Input: part model. Units: mm. Frame: model coordinates. A direction names the side the tool comes from. Coordinates: 2 decimals unless noted, no trailing zeros. Write each loop counter-clockwise with the first axis right and the second up, starting at its lowest first coordinate (ties: lowest second). Pieces come first, ordered by that corner, then holes.
from build123d import *

# Parameters (mm, degrees)
F1_DEPTH = 38.1
F3_DEPTH = 25
F5_R     = 4.7625
F6_DEPTH = 34.1
F8_DEPTH = 34.1
F9_DEPTH = 50


with BuildPart() as f1:
    # F0 (on Top) → F1 (new body)
    with BuildSketch(Plane.XY):
        Polygon((23.88, 22.062646), (-14.22, 22.062646), (-14.22, 3.012646), (-14.22, -16.037354), (23.88, -16.037354), align=None)
        with BuildLine():
            ThreePointArc((9.5925, 3.012646), (4.83, -1.749854), (0.0675, 3.012646))
            ThreePointArc((0.0675, 3.012646), (4.83, 7.775146), (9.5925, 3.012646))
        make_face(mode=Mode.SUBTRACT)
    extrude(amount=F1_DEPTH)

    # F2 (on face) → F3 (cut)
    with BuildSketch(Plane.YZ.offset(23.88)):
        with BuildLine():
            ThreePointArc((-1.749854, 19.05), (3.012646, 14.2875), (7.775146, 19.05))
            ThreePointArc((7.775146, 19.05), (3.012646, 23.8125), (-1.749854, 19.05))
        make_face()
    extrude(amount=-F3_DEPTH, mode=Mode.SUBTRACT)

    # F5 (on face) → F6 (cut)
    with BuildSketch(Plane.XY.offset(38.1)):
        Polygon((19.88, 18.062646), (4.83, 18.062646), (-10.22, 18.062646), (-10.22, 3.012646), (-10.22, -12.037354), (4.83, -12.037354), (19.88, -12.037354), (19.88, 3.012646), align=None)
        with Locations((4.83, 3.012646)):
            Circle(F5_R, mode=Mode.SUBTRACT)
    extrude(amount=-F6_DEPTH, mode=Mode.SUBTRACT)

    # F7 (on face) → F8 (cut)
    with BuildSketch(Plane(origin=(-14.22, 0, 0), x_dir=(0, -1, 0), z_dir=(-1, 0, 0))):
        Polygon((12.037354, 34.1), (-3.012646, 34.1), (-18.062646, 34.1), (-18.062646, 19.05), (-18.062646, 4), (-3.012646, 4), (12.037354, 4), (12.037354, 19.05), align=None)
    extrude(amount=-F8_DEPTH, mode=Mode.SUBTRACT)

    # F4 (on face) → F9 (cut)
    with BuildSketch(Plane.XZ.offset(16.037354)):
        Polygon((-14.22, 0), (23.88, 38.1), (-14.22, 38.1), align=None)
    extrude(amount=-F9_DEPTH, mode=Mode.SUBTRACT)


solid = f1.part
Item 1: Section query C-C, the plane z = 8.5. Return loops of the section in (x, y).
Item 2: Section query B-B, the plane x = 4.83. Return loops of the section in (y, z), then the cut area to 3 significant figures.
Item 3: Section query A-A, the plane z = 19.05. Return loops of the section in (x, y), then the cut area to 3 significant figures.
Item 4: Section query D-D, the plane y = 1. Return loops of the section in (x, z), then the cut area to 3 significant figures.
Item 5: Access query for faces 1 (the face through (23.88, -1, 23)), 2 (the face through (1, 7, 4)). Directions: +Z, -Z, +X, -X, +Y, -Y. A direction counts if a zero-diameter tool reaches every point of the face in a straight line with its end or side. Return the directions, or none.
Item 6: Pull-direction query (X, two-part tool) for faces 3 (the face through (5.862, -1.637, 1.972)), 4 (the face through (13, -16.037, 10)), 5 (the face through (19.88, -1, 23)); classes: released by +X, released by -X, zero draft, split by the parting line, or undercut.
Item 7: Material intervals for line 1 (Y direction, x = 18, z = 31.5); line 2 (Y direction, x = 4.83, z = 3.25); line 3 (Z direction, x = 19.5, y = 1.5), sorted ascending.
Item 8: Pin query (flat end, axial travel): pin 1 Ø15 at (x, y) = (4.83, 3.01) entering from +Z; pin 2 Ø10 at (x, z) = (-10, 7) entering from -Y; pin 3 Ø15 at (y, z) = (10.5, 26) entering from -X. Return the tip coordinate at first contact, or that it passes through.
The answers:
1. outline: (-5.72, -16.04) - (23.88, -16.04) - (23.88, 22.06) - (-5.72, 22.06) - (-5.72, 18.06) - (19.88, 18.06) - (19.88, -12.04) - (-5.72, -12.04) - close
2. outline: (-16.04, 0) - (-1.75, 0) - (-1.75, 4) - (-12.04, 4) - (-12.04, 19.05) - (-16.04, 19.05) - close; (7.78, 0) - (22.06, 0) - (22.06, 19.05) - (18.06, 19.05) - (18.06, 4) - (7.78, 4) - close
2. area: 235 mm2
3. outline: (4.83, -16.04) - (23.88, -16.04) - (23.88, -1.75) - (19.88, -1.75) - (19.88, -12.04) - (4.83, -12.04) - close; (4.83, 18.06) - (19.88, 18.06) - (19.88, 7.78) - (23.88, 7.78) - (23.88, 22.06) - (4.83, 22.06) - close
3. area: 235 mm2
4. outline: (-14.22, 0) - (0.51, 0) - (0.51, 4) - (-10.22, 4) - close; (9.15, 0) - (23.88, 0) - (23.88, 14.73) - (19.88, 14.73) - (19.88, 4) - (9.15, 4) - close; (19.88, 23.37) - (23.88, 23.37) - (23.88, 38.1) - (19.88, 34.1) - close
4. area: 204 mm2
5. face 1: +Z, -Z, +X, +Y, -Y
5. face 2: +Z, -X
6. face 3: undercut
6. face 4: zero draft
6. face 5: released by -X
7. line 1: y = -16.04 to -12.04, 18.06 to 22.06
7. line 2: y = -16.04 to -1.75, 7.78 to 22.06
7. line 3: z = 0 to 4
8. pin 1: stops at z = 4
8. pin 2: stops at y = -16.04
8. pin 3: stops at x = 19.88
